```python
from build123d import *

# Parameters (mm, degrees)
SKETCH1_R           = 6.3246
SKETCH1_R_2         = 4.6736
BOSS_EXTRUDE1_DEPTH = 24.84755
SKETCH2_W           = 0.9652
SKETCH2_H           = 1.143
CHAMFER1_SIZE       = 0.889


with BuildPart() as part:
    # Sketch1 → Boss-Extrude1 (new body, symmetric)
    with BuildSketch(Plane.XY):
        Circle(SKETCH1_R)
        Circle(SKETCH1_R_2, mode=Mode.SUBTRACT)
    extrude(amount=BOSS_EXTRUDE1_DEPTH, both=True)

    # Sketch2 → Cut-Revolve1 (revolve, cut)
    with BuildSketch(Plane(origin=(0, 0, 0), x_dir=(1, 0, 0), z_dir=(0, 1, 0))):
        with Locations((5.842, 21.73605)):
            Rectangle(SKETCH2_W, SKETCH2_H)
    cut_revolve1 = revolve(axis=Axis((0, 0, 1000), (0, 0, -1)), mode=Mode.SUBTRACT)

    # Mirror1: Cut-Revolve1 across plane
    add(cut_revolve1.mirror(Plane.XY), mode=Mode.SUBTRACT)

    # Chamfer1
    chamfer1_edges = [part.edges().sort_by_distance(p)[0] for p in [
        (-6.3246, 0, -24.84755),
        (-6.3246, 0, 24.84755),
    ]]
    chamfer(chamfer1_edges, length=CHAMFER1_SIZE)


solid = part.part
```
Here's how the part is built. I have some questions about the finished solid (model axes, mm). A direction names the side the tool comes from. Round coordinates to 2 decimals unless told otherwise and drop trailing zeros. Loops run counter-clockwise (first coordinate to the right, second up) from the corner with the lowest first, then second, coordinate; pieces in that order, holes last. Notation, with made-up numbers: (-0.5, 39) -> (7.5, 39) arc R8 ccw to (7.5, 43) -> close; hole circle Ø2 at (72, 65.5). An arc over 180 degrees is marked (long way). Answer as CSV lines item,"result".
1. For pin 1 (4 mm diameter, centred on x = -3, z = -3, fed in from +Y), with a flat end and sliding along its axis, tell me the tip position at first contact or that it passes through.
Final values:
pin 1,"stops at y = 6.25"
2. If we section it at C-C on z = -1.5: Please give me the cut outline in (x, y), plus the area to 3 significant figures.
Final values:
outline,"circle Ø12.65 at (0, 0); hole circle Ø9.35 at (0, 0)"
area,"57.0 mm^2"
3. If we section it at A-A on x = 0: Please give me the cut outline in (y, z).
Final values:
outline,"(-6.32, -23.96) -> (-5.44, -24.85) -> (-4.67, -24.85) -> (-4.67, 24.85) -> (-5.44, 24.85) -> (-6.32, 23.96) -> (-6.32, 22.31) -> (-5.36, 22.31) -> (-5.36, 21.16) -> (-6.32, 21.16) -> (-6.32, -21.16) -> (-5.36, -21.16) -> (-5.36, -22.31) -> (-6.32, -22.31) -> close; (4.67, -24.85) -> (5.44, -24.85) -> (6.32, -23.96) -> (6.32, -22.31) -> (5.36, -22.31) -> (5.36, -21.16) -> (6.32, -21.16) -> (6.32, 21.16) -> (5.36, 21.16) -> (5.36, 22.31) -> (6.32, 22.31) -> (6.32, 23.96) -> (5.44, 24.85) -> (4.67, 24.85) -> close"
4. Which directions (+Z, -Z, +X, -X, +Y, -Y) give clear straight access to the entire face, cutting with the end or side of a thin tool? Please do faces 1 (the face through (5, -3, 21.165)), 2 (the face through (6, 2, 0)).
Final values:
face 1,"none"
face 2,"+Z, -Z"
5. If I drill on L1, parallel to Y at x = 0, z = 14.5; L2, parallel to Z at x = 3.75, y = -5; L3, parallel to Y at x = -2.5, z = -10, over which ranges is the centre line in solid material (lowest first)?
Final values:
L1,"y = -6.32 to -4.67, 4.67 to 6.32"
L2,"z = -24.03 to -22.31, -21.16 to 21.16, 22.31 to 24.03"
L3,"y = -5.81 to -3.95, 3.95 to 5.81"
6. Thinking about a two-plate mould opening in Y: for faces 3 (the face through (4.46, 1.4, -0.35)), 4 (the face through (6, 2, -23)), 5 (the face through (5, -3, -22.308)), which applies, released by +Y, released by -Y, zero draft, split by the parting line, or undercut?
Final values:
face 3,"undercut"
face 4,"split by the parting line"
face 5,"zero draft"
